Verification items for the finished model (mm, model axes). A direction names the side the tool comes from. Give positions to 0.01 mm unless a question says otherwise; leave off trailing zeros. Order: outer loops, then holes, each group sorted by start corner. A loop starts at its lowest first (then second) coordinate and runs counter-clockwise, first axis right, second up. Notation, with made-up numbers: (-29, -4.75) - (-22, -4.75) arc R19 cw to (-22, 32.25) - close; hole circle Ø7 at (63.5, -38). An arc over 180 degrees is marked (long way). Answer as a JSON object with one key per item and string values.
```python
from build123d import *

# Parameters (mm, degrees)
SALIENTE_EXTRUIR1_DEPTH = 7
CROQUIS2_7_W            = 8
CROQUIS2_7_H            = 25
CROQUIS2_7_W_2          = 25
CROQUIS2_7_H_2          = 8
SALIENTE_EXTRUIR3_DEPTH = 27
SALIENTE_EXTRUIR5_DEPTH = 37
CROQUIS10_R             = 1.9
CORTAR_EXTRUIR3_DEPTH   = 22
CROQUIS11_R             = 3.1
CORTAR_EXTRUIR4_DEPTH   = 6
CORTAR_EXTRUIR5_DEPTH   = 6
CORTAR_EXTRUIR6_START   = -7
CROQUIS17_W             = 8
CROQUIS17_H             = 11.32382093
CORTAR_EXTRUIR6_DEPTH   = 7
CROQUIS17_4_W           = 8
CROQUIS17_4_H           = 11.32382093
CORTAR_EXTRUIR7_DEPTH   = 20
CROQUIS17_5_W           = 48
CROQUIS17_5_H           = 5
SALIENTE_EXTRUIR6_DEPTH = 16
CORTAR_EXTRUIR8_DEPTH   = 10


with BuildPart() as part:
    # Croquis2 → Saliente-Extruir1 (new body)
    with BuildSketch(Plane.XY):
        with BuildLine():
            Line((-47.286620614, 40.816010109), (-47.286620614, -49.183989891))
            ThreePointArc((-47.286620614, -49.183989891), (-45.236368082, -54.133737359), (-40.286620614, -56.183989891))
            Line((-40.286620614, -56.183989891), (3.713379386, -56.183989891))
            ThreePointArc((3.713379386, -56.183989891), (8.663126854, -54.133737359), (10.713379386, -49.183989891))
            Line((10.713379386, -49.183989891), (10.713379386, 40.816010109))
            Line((10.713379386, 40.816010109), (-47.286620614, 40.816010109))
        make_face()
    extrude(amount=SALIENTE_EXTRUIR1_DEPTH)

    # Croquis2_7 → Saliente-Extruir3 (add)
    with BuildSketch(Plane.XY):
        with Locations((14.713379386, 7.316010109)):
            Rectangle(CROQUIS2_7_W, CROQUIS2_7_H)
        Polygon((10.713379386, 40.816010109), (-5.786620614, 40.816010109), (-5.786620614, 48.816010109), (18.713379386, 48.816010109), (18.713379386, 19.816010109), (10.713379386, 19.816010109), align=None)
        with Locations((-18.286620614, 44.816010109)):
            Rectangle(CROQUIS2_7_W_2, CROQUIS2_7_H_2)
        Polygon((-47.286620614, 19.816010109), (-47.286620614, 40.816010109), (-30.786620614, 40.816010109), (-30.786620614, 48.816010109), (-55.286620614, 48.816010109), (-55.286620614, 19.816010109), align=None)
        with Locations((-51.286620614, 7.316010109)):
            Rectangle(CROQUIS2_7_W, CROQUIS2_7_H)
    extrude(amount=SALIENTE_EXTRUIR3_DEPTH)

    # Croquis2_14 → Saliente-Extruir5 (add)
    with BuildSketch(Plane.XY):
        with BuildLine():
            ThreePointArc((-19.286620614, 91.616010109), (-18.286620614, 83.539831039), (-17.286620614, 91.616010109))
            Line((-17.286620614, 91.616010109), (-17.286620614, 103.616010109))
            Line((-17.286620614, 103.616010109), (-7.286620614, 103.616010109))
            Line((-7.286620614, 103.616010109), (-7.286620614, 74.616010109))
            Line((-7.286620614, 74.616010109), (18.713379386, 48.816010109))
            Line((18.713379386, 48.816010109), (-5.786620614, 48.816010109))
            Line((-5.786620614, 48.816010109), (-30.786620614, 48.816010109))
            Line((-30.786620614, 48.816010109), (-55.286620614, 48.816010109))
            Line((-55.286620614, 48.816010109), (-29.286620614, 74.616010109))
            Line((-29.286620614, 74.616010109), (-29.286620614, 103.616010109))
            Line((-29.286620614, 103.616010109), (-19.286620614, 103.616010109))
            Line((-19.286620614, 103.616010109), (-19.286620614, 91.616010109))
        make_face()
    extrude(amount=SALIENTE_EXTRUIR5_DEPTH)

    # Croquis10 → Cortar-Extruir3 (cut)
    with BuildSketch(Plane(origin=(-7.286620614, 0, 0), x_dir=(0, 0, -1), z_dir=(1, 0, 0))):
        with Locations((-9, 94.816010109)):
            Circle(CROQUIS10_R)
        with Locations((-18, 94.816010109)):
            Circle(CROQUIS10_R)
        with Locations((-27, 94.816010109)):
            Circle(CROQUIS10_R)
    extrude(amount=-CORTAR_EXTRUIR3_DEPTH, mode=Mode.SUBTRACT)

    # Croquis11 → Cortar-Extruir4 (cut)
    with BuildSketch(Plane(origin=(-7.286620614, 0, 0), x_dir=(0, 0, -1), z_dir=(1, 0, 0))):
        with Locations((-27, 94.816010109)):
            Circle(CROQUIS11_R)
        with Locations((-18, 94.816010109)):
            Circle(CROQUIS11_R)
        with Locations((-9, 94.816010109)):
            Circle(CROQUIS11_R)
    extrude(amount=-CORTAR_EXTRUIR4_DEPTH, mode=Mode.SUBTRACT)

    # Croquis12 → Cortar-Extruir5 (cut)
    with BuildSketch(Plane.ZY.offset(29.286620614)):
        Polygon((21.233161507, 94.816010109), (19.616580754, 97.616010109), (16.383419246, 97.616010109), (14.766838493, 94.816010109), (16.383419246, 92.016010109), (19.616580754, 92.016010109), align=None)
        Polygon((12.233161507, 94.816010109), (10.616580754, 97.616010109), (7.383419246, 97.616010109), (5.766838493, 94.816010109), (7.383419246, 92.016010109), (10.616580754, 92.016010109), align=None)
        Polygon((30.233161507, 94.816010109), (28.616580754, 97.616010109), (25.383419246, 97.616010109), (23.766838493, 94.816010109), (25.383419246, 92.016010109), (28.616580754, 92.016010109), align=None)
    extrude(amount=-CORTAR_EXTRUIR5_DEPTH, mode=Mode.SUBTRACT)

    # Croquis17 → Cortar-Extruir6 (cut)
    with BuildSketch(Plane.XY.offset(7).offset(CORTAR_EXTRUIR6_START)):
        with BuildLine():
            Line((10.713379386, -5.183989891), (-18.286620614, -5.183989891))
            Line((-18.286620614, -5.183989891), (-47.286620614, -5.183989891))
            Line((-47.286620614, -5.183989891), (-47.286620614, -49.183989891))
            ThreePointArc((-47.286620614, -49.183989891), (-45.236368082, -54.133737359), (-40.286620614, -56.183989891))
            Line((-40.286620614, -56.183989891), (3.713379386, -56.183989891))
            ThreePointArc((3.713379386, -56.183989891), (8.663126854, -54.133737359), (10.713379386, -49.183989891))
            Line((10.713379386, -49.183989891), (10.713379386, -5.183989891))
        make_face()
        Polygon((-18.286620614, -5.183989891), (-18.286620614, -0.860168961), (-42.286620614, -0.860168961), (-42.286620614, 6.139831039), (-47.286620614, 6.139831039), (-47.286620614, -5.183989891), align=None)
        Polygon((5.713379386, -0.860168961), (-18.286620614, -0.860168961), (-18.286620614, -5.183989891), (10.713379386, -5.183989891), (10.713379386, 6.139831039), (5.713379386, 6.139831039), align=None)
        Polygon((-18.286620614, 6.139831039), (-18.286620614, 2.639831039), (-18.286620614, -0.860168961), (5.713379386, -0.860168961), (5.713379386, 6.139831039), align=None)
        Polygon((-18.286620614, -0.860168961), (-18.286620614, 2.639831039), (-18.286620614, 6.139831039), (-42.286620614, 6.139831039), (-42.286620614, -0.860168961), align=None)
        with Locations((-51.286620614, 0.477920574)):
            Rectangle(CROQUIS17_W, CROQUIS17_H)
        with Locations((14.713379386, 0.477920574)):
            Rectangle(CROQUIS17_W, CROQUIS17_H)
    extrude(amount=CORTAR_EXTRUIR6_DEPTH, mode=Mode.SUBTRACT)

    # Croquis17_4 → Cortar-Extruir7 (cut)
    with BuildSketch(Plane.XY.offset(7)):
        with Locations((-51.286620614, 0.477920574)):
            Rectangle(CROQUIS17_4_W, CROQUIS17_4_H)
        with Locations((14.713379386, 0.477920574)):
            Rectangle(CROQUIS17_4_W, CROQUIS17_4_H)
    extrude(amount=CORTAR_EXTRUIR7_DEPTH, mode=Mode.SUBTRACT)

    # Croquis17_5 → Saliente-Extruir6 (add)
    with BuildSketch(Plane.XY.offset(7)):
        with Locations((-18.286620614, 8.639831039)):
            Rectangle(CROQUIS17_5_W, CROQUIS17_5_H)
    extrude(amount=SALIENTE_EXTRUIR6_DEPTH)

    # Croquis18 → Cortar-Extruir8 (cut)
    with BuildSketch(Plane.XZ.offset(-6.139831039)):
        with BuildLine():
            ThreePointArc((-27.286620614, 17), (-26.225960442, 17.439339828), (-25.786620614, 18.5))
            Line((-25.786620614, 18.5), (-27.286620614, 18.5))
            Line((-27.286620614, 18.5), (-27.286620614, 17))
        make_face()
        with BuildLine():
            Line((-27.286620614, 18.5), (-25.786620614, 18.5))
            ThreePointArc((-25.786620614, 18.5), (-28.347280786, 19.560660172), (-27.286620614, 17))
            Line((-27.286620614, 17), (-27.286620614, 18.5))
        make_face()
        with BuildLine():
            ThreePointArc((-7.786620614, 18.5), (-9.286620614, 20), (-10.786620614, 18.5))
            Line((-10.786620614, 18.5), (-9.286620614, 18.5))
            Line((-9.286620614, 18.5), (-9.286620614, 17))
            ThreePointArc((-9.286620614, 17), (-8.225960442, 17.439339828), (-7.786620614, 18.5))
        make_face()
        with BuildLine():
            Line((-9.286620614, 18.5), (-10.786620614, 18.5))
            ThreePointArc((-10.786620614, 18.5), (-10.347280786, 17.439339828), (-9.286620614, 17))
            Line((-9.286620614, 17), (-9.286620614, 18.5))
        make_face()
        with BuildLine():
            ThreePointArc((-9.286620614, 13), (-10.347280786, 12.560660172), (-10.786620614, 11.5))
            Line((-10.786620614, 11.5), (-9.286620614, 11.5))
            Line((-9.286620614, 11.5), (-9.286620614, 13))
        make_face()
        with BuildLine():
            Line((-9.286620614, 11.5), (-10.786620614, 11.5))
            ThreePointArc((-10.786620614, 11.5), (-9.286620614, 10), (-7.786620614, 11.5))
            ThreePointArc((-7.786620614, 11.5), (-8.225960442, 12.560660172), (-9.286620614, 13))
            Line((-9.286620614, 13), (-9.286620614, 11.5))
        make_face()
        with BuildLine():
            ThreePointArc((-27.286620614, 13), (-28.347280786, 10.439339828), (-25.786620614, 11.5))
            Line((-25.786620614, 11.5), (-27.286620614, 11.5))
            Line((-27.286620614, 11.5), (-27.286620614, 13))
        make_face()
        with BuildLine():
            Line((-27.286620614, 11.5), (-25.786620614, 11.5))
            ThreePointArc((-25.786620614, 11.5), (-26.225960442, 12.560660172), (-27.286620614, 13))
            Line((-27.286620614, 13), (-27.286620614, 11.5))
        make_face()
    extrude(amount=-CORTAR_EXTRUIR8_DEPTH, mode=Mode.SUBTRACT)


solid = part.part
```
(1) Gauge pin test, flat ends, axial feed: pin 1 Ø5 at (y, z) = (94.82, 27) entering from -X; pin 2 Ø8 at (y, z) = (83, 19) entering from +X; pin 3 Ø8 at (x, z) = (8, 25) entering from +Y; pin 4 Ø2.5 at (y, z) = (94.82, 9) entering from +X. Record the tip position at first contact, or that the pin passes through.
Computed values:
{"pin 1": "stops at x = -23.29", "pin 2": "stops at x = -7.29", "pin 3": "stops at y = 63.42", "pin 4": "passes through"}
(2) Access from +Z, -Z, +X, -X, +Y, -Y to the whole of each face (thin tool, end or side, straight path). Record for faces 4 (the flat face through (-19, 42, 27)), 5 (the flat face through (-47.287, 23, 17)), 6 (the flat face through (-23.287, 97, 27)).
Computed values:
{"face 4": "+Z, +X, -X, -Y", "face 5": "+Z, -Y", "face 6": "-X"}
(3) Section check B-B (y = 37.5). Record the cut outline in (x, z).
Computed values:
{"outline": "(-55.29, 0) - (18.71, 0) - (18.71, 27) - (10.71, 27) - (10.71, 7) - (-47.29, 7) - (-47.29, 27) - (-55.29, 27) - close"}
(4) Section check A-A (z = 2). Record the cut outline in (x, y).
Computed values:
{"outline": "(-55.29, 6.14) - (18.71, 6.14) - (18.71, 48.82) - (-7.29, 74.62) - (-7.29, 103.62) - (-17.29, 103.62) - (-17.29, 91.62) arc R4.1 cw (long way) to (-19.29, 91.62) - (-19.29, 103.62) - (-29.29, 103.62) - (-29.29, 74.62) - (-55.29, 48.82) - close"}
(5) Section check C-C (x = -34.5). Record the cut outline in (y, z), then the cut area to 3 significant figures.
Computed values:
{"outline": "(6.14, 0) - (69.44, 0) - (69.44, 37) - (48.82, 37) - (48.82, 27) - (40.82, 27) - (40.82, 7) - (11.14, 7) - (11.14, 23) - (6.14, 23) - close", "area": "1,300 mm²"}
(6) Material ranges on line 1 along X through (y, z) = (8.9, 11.5); line 2 along Y through (x, z) = (-11.7, 18); line 3 along X through (y, z) = (97, 19), recorded low to high. Write a range as [from, to].
Computed values:
{"line 1": "x = [-55.29, -47.29], [-42.29, -28.79], [-25.79, -10.79], [-7.79, 5.71], [10.71, 18.71]", "line 2": "y = [6.14, 11.14], [40.82, 91.72], [97.92, 103.62]", "line 3": "x = [-23.29, -19.29], [-17.29, -13.29]"}
(7) Release check for a two-part mould opening along Z. For faces 1 (the flat face through (-19, 40.816, 17)), 2 (the flat face through (-18, 71, 37)), 3 (the flat face through (-26, 97.616, 18)) record: pulls with the +Z half, pulls with the -Z half, needs draft (parallel to the pull), parting line crosses it, or undercut.
Computed values:
{"face 1": "needs draft", "face 2": "pulls with the +Z half", "face 3": "undercut"}
(8) Section check D-D (y = 82). Record the cut outline in (x, z), then the cut area to 3 significant figures.
Computed values:
{"outline": "(-29.29, 0) - (-7.29, 0) - (-7.29, 37) - (-29.29, 37) - close", "area": "814 mm²"}
